from build123d import *

# Parameters (mm, degrees)
BASE_EXTRUDE_DEPTH  = 12.7
BOSS_EXTRUDE1_DEPTH = 12.7


with BuildPart() as part:
    # Sketch1 → Base-Extrude (new, symmetric)
    with BuildSketch(Plane.XY):
        with BuildLine():
            Line((-20.6375, 19.1389), (-20.6375, 11.29515134))
            ThreePointArc((-20.6375, 11.29515134), (-19.1389, 8.6995), (-20.6375, 6.10384866))
            Line((-20.6375, 6.10384866), (-20.6375, 1.4986))
            ThreePointArc((-20.6375, 1.4986), (-20.198570222, 0.438929778), (-19.1389, 0))
            Line((-19.1389, 0), (19.1389, 0))
            ThreePointArc((19.1389, 0), (20.198570222, 0.438929778), (20.6375, 1.4986))
            Line((20.6375, 1.4986), (20.6375, 6.10384866))
            ThreePointArc((20.6375, 6.10384866), (19.1389, 8.6995), (20.6375, 11.29515134))
            Line((20.6375, 11.29515134), (20.6375, 19.1389))
            ThreePointArc((20.6375, 19.1389), (20.198570222, 20.198570222), (19.1389, 20.6375))
            Line((19.1389, 20.6375), (12.6111, 20.6375))
            ThreePointArc((12.6111, 20.6375), (11.551429778, 20.198570222), (11.1125, 19.1389))
            Line((11.1125, 19.1389), (11.1125, 14.2875))
            Line((11.1125, 14.2875), (12.6111, 14.2875))
            Line((12.6111, 14.2875), (12.6111, 19.1389))
            Line((12.6111, 19.1389), (19.1389, 19.1389))
            Line((19.1389, 19.1389), (19.1389, 12.050471471))
            ThreePointArc((19.1389, 12.050471471), (17.6403, 8.6995), (19.1389, 5.348528529))
            Line((19.1389, 5.348528529), (19.1389, 1.4986))
            Line((19.1389, 1.4986), (-19.1389, 1.4986))
            Line((-19.1389, 1.4986), (-19.1389, 5.348528529))
            ThreePointArc((-19.1389, 5.348528529), (-17.6403, 8.6995), (-19.1389, 12.050471471))
            Line((-19.1389, 12.050471471), (-19.1389, 19.1389))
            Line((-19.1389, 19.1389), (-12.6111, 19.1389))
            Line((-12.6111, 19.1389), (-12.6111, 14.2875))
            Line((-12.6111, 14.2875), (-11.1125, 14.2875))
            Line((-11.1125, 14.2875), (-11.1125, 19.1389))
            ThreePointArc((-11.1125, 19.1389), (-11.551429778, 20.198570222), (-12.6111, 20.6375))
            Line((-12.6111, 20.6375), (-19.1389, 20.6375))
            ThreePointArc((-19.1389, 20.6375), (-20.198570222, 20.198570222), (-20.6375, 19.1389))
        make_face()
    base_extrude = extrude(amount=BASE_EXTRUDE_DEPTH, both=True)

    # Mirror1: Base-Extrude across plane
    add(base_extrude.mirror(Plane.ZX))

    # Sketch2 → Boss-Extrude1 (add, symmetric)
    with BuildSketch(Plane(origin=(20.16125, 0.15875, 0), x_dir=(0, -1, 0), z_dir=(0, 0, 1))):
        with BuildLine():
            Line((-20.47875, 19.61515), (-20.47875, 11.77140134))
            ThreePointArc((-20.47875, 11.77140134), (-18.98015, 9.17575), (-20.47875, 6.58009866))
            Line((-20.47875, 6.58009866), (-20.47875, 1.97485))
            ThreePointArc((-20.47875, 1.97485), (-20.039820222, 0.915179778), (-18.98015, 0.47625))
            Line((-18.98015, 0.47625), (19.29765, 0.47625))
            ThreePointArc((19.29765, 0.47625), (20.357320222, 0.915179778), (20.79625, 1.97485))
            Line((20.79625, 1.97485), (20.79625, 6.58009866))
            ThreePointArc((20.79625, 6.58009866), (19.29765, 9.17575), (20.79625, 11.77140134))
            Line((20.79625, 11.77140134), (20.79625, 19.61515))
            ThreePointArc((20.79625, 19.61515), (20.357320222, 20.674820222), (19.29765, 21.11375))
            Line((19.29765, 21.11375), (12.76985, 21.11375))
            ThreePointArc((12.76985, 21.11375), (11.710179778, 20.674820222), (11.27125, 19.61515))
            Line((11.27125, 19.61515), (11.27125, 14.76375))
            Line((11.27125, 14.76375), (12.76985, 14.76375))
            Line((12.76985, 14.76375), (12.76985, 19.61515))
            Line((12.76985, 19.61515), (19.29765, 19.61515))
            Line((19.29765, 19.61515), (19.29765, 12.526721471))
            ThreePointArc((19.29765, 12.526721471), (17.79905, 9.17575), (19.29765, 5.824778529))
            Line((19.29765, 5.824778529), (19.29765, 1.97485))
            Line((19.29765, 1.97485), (-18.98015, 1.97485))
            Line((-18.98015, 1.97485), (-18.98015, 5.824778529))
            ThreePointArc((-18.98015, 5.824778529), (-17.48155, 9.17575), (-18.98015, 12.526721471))
            Line((-18.98015, 12.526721471), (-18.98015, 19.61515))
            Line((-18.98015, 19.61515), (-12.45235, 19.61515))
            Line((-12.45235, 19.61515), (-12.45235, 14.76375))
            Line((-12.45235, 14.76375), (-10.95375, 14.76375))
            Line((-10.95375, 14.76375), (-10.95375, 19.61515))
            ThreePointArc((-10.95375, 19.61515), (-11.392679778, 20.674820222), (-12.45235, 21.11375))
            Line((-12.45235, 21.11375), (-18.98015, 21.11375))
            ThreePointArc((-18.98015, 21.11375), (-20.039820222, 20.674820222), (-20.47875, 19.61515))
        make_face()
    boss_extrude1 = extrude(amount=BOSS_EXTRUDE1_DEPTH, both=True)

    # Mirror2: Boss-Extrude1 across plane
    add(boss_extrude1.mirror(Plane(origin=(0, 0, 0), x_dir=(0, 0, 1), z_dir=(1, 0, 0))))


solid = part.part
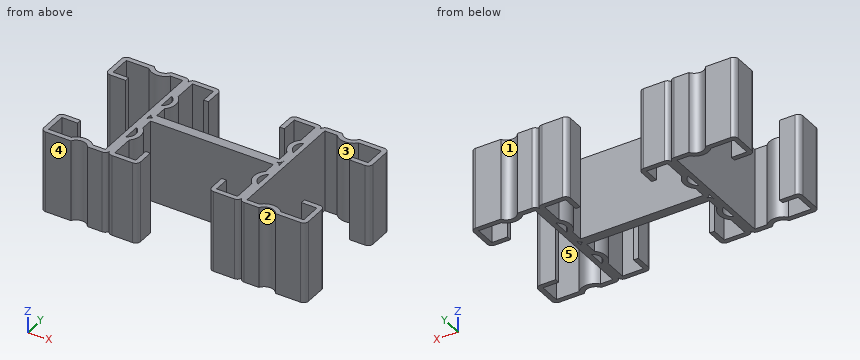
Work out the finished part from the listing and answer in its coordinate system (mm). Face numbers are marked on the shaded views. A direction names the side the tool comes from. Coordinates: 2 decimals unless noted, no trailing zeros. Write each loop counter-clockwise with the first axis right and the second up, starting at its lowest first coordinate (ties: lowest second). Pieces come first, ordered by that corner, then holes. Notation, with made-up numbers: M 77,83 L 91,83 A17 cw 91,104 Z; hole C 35,-3 d10. An arc over 180 degrees is marked long. Use one line per item in the form item = value. Start each with the question number.
1. Each of these flat-tipped pins is pushed along its axis until it touches: P1, Ø5, axis at y = -1, z = -7.5, coming from the -X side; P2, Ø1.2, axis at y = 11.5, z = -0.5, coming from the -X side; P3, Ø4, axis at y = -10.5, z = 7, coming from the +X side. Where does it stop, or does it pass through?
2. The part is cut by section A-A (x = 16.5). Give the vertices of the cut face in (y, z), plus the area to 3 significant figures.
3. The part is cut by section D-D (y = 7.5). Give the vertices of the cut face in (x, z).
4. Straight lines are drawn through the part: probe 1 along X at (y, z) = (-14, 6) (3 decimals); probe 2 along X at (y, z) = (15, -1.5) (1 decimal); probe 3 along X at (y, z) = (-12.5, -5) (3 decimals). For each, find the intervals that lie inside material, in ascending order. Write a range as from..to.
5. The mould has two halves that part along Y. Classify the marked faces 1, 2 and 3: released by +Y, released by -Y, zero draft, split by the parting line, or undercut.
6. A tool of negligible diameter and unlimited length cuts with its end or side. For the marked faces 4 and 5, from which of +Z, -Z, +X, -X, +Y, -Y can it reach the whole face along a straight path? Write none if from no direction.
7. The part is cut by section C-C (z = 1). Give the number of separate pieces and of enclosed holes in the cut face, plus the area to 3 significant figures.
8. The part is cut by section B-B (y = 3). Give the vertices of the cut face in (x, z), plus the area to 3 significant figures.
Evaluation:
q1.P1 = -22.14
q1.P2 = -41.19
q1.P3 = 41.27
q2.outline = M -20.64,-12.7 L -19.14,-12.7 L -19.14,12.7 L -20.64,12.7 Z; M -1.5,-12.7 L 1.5,-12.7 L 1.5,12.7 L -1.5,12.7 Z; M 19.14,-12.7 L 20.64,-12.7 L 20.64,12.7 L 19.14,12.7 Z
q2.area = 152 mm^2
q3.outline = M -22.14,-12.7 L -20.64,-12.7 L -20.64,12.7 L -22.14,12.7 Z; M -19.39,-12.7 L -17.8,-12.7 L -17.8,12.7 L -19.39,12.7 Z; M 17.8,-12.7 L 19.39,-12.7 L 19.39,12.7 L 17.8,12.7 Z; M 20.64,-12.7 L 22.14,-12.7 L 22.14,12.7 L 20.64,12.7 Z
q4.probe_1 = -41.275..-39.776, -22.136..-19.139, 19.139..22.136, 39.776..41.275
q4.probe_2 = -41.3..-39.8, -22.1..-19.1, -12.6..-11.1, 11.1..12.6, 19.1..22.1, 39.8..41.3
q4.probe_3 = -41.271..-34.925, -22.136..-19.139, 19.139..22.136, 34.925..41.271
q5.face_1 = released by +Y
q5.face_2 = released by -Y
q5.face_3 = undercut
q6.face_4 = +Z, -Z, +X, -X, -Y
q6.face_5 = +Z, -Z
q7.separate_pieces = 1
q7.enclosed_holes = 6
q7.area = 631 mm^2
q8.outline = M -22.14,-12.7 L -19.14,-12.7 L -19.14,12.7 L -22.14,12.7 Z; M 19.14,-12.7 L 22.14,-12.7 L 22.14,12.7 L 19.14,12.7 Z
q8.area = 152 mm^2
